Part model, mm, in its own coordinate system. Face numbers are marked on the shaded views. A direction names the side the tool comes from. Coordinates: 2 decimals unless noted, no trailing zeros. Order: outer loops, then holes, each group sorted by start corner. A loop starts at its lowest first (then second) coordinate and runs counter-clockwise, first axis right, second up. Notation, with made-up numbers: M -0.75,-36 L 46.25,-36 A7 ccw 46.25,-31 Z; hole C 60.25,35.5 d3. An arc over 180 degrees is marked long. Answer in a Markdown table with one row per item. Add a question column.
from build123d import *

# Parameters (mm, degrees)
F1_DEPTH  = 67
F2_W      = 19
F2_H      = 59.602782
F3_DEPTH  = 45
F4_W      = 19
F4_H      = 59.070988
F5_DEPTH  = 45
F7_DEPTH  = 19
F9_DEPTH  = 19
F10_W     = 28
F10_H     = 14.292508
F11_DEPTH = 66.9
F13_DEPTH = 14.4
F14_R     = 12.5
F15_DEPTH = 65.5


with BuildPart() as f1:
    # F0 (on Front) → F1 (new body)
    with BuildSketch(Plane.XZ):
        Polygon((0, 20), (0, 0), (63, 0), (63, 75), (0, 75), (0, 55), (38, 55), (38, 20), align=None)
    extrude(amount=F1_DEPTH)

    # F2 (on face) → F3 (join)
    with BuildSketch(Plane.YZ.offset(63)):
        with Locations((-49.5, 37.198609)):
            Rectangle(F2_W, F2_H)
    extrude(amount=F3_DEPTH)

    # F4 (on face) → F5 (join)
    with BuildSketch(Plane.YZ.offset(63)):
        with Locations((-16.24, 37.464506)):
            Rectangle(F4_W, F4_H)
    extrude(amount=F5_DEPTH)

    # F6 (on face) → F7 (join)
    with BuildSketch(Plane.XZ.offset(59)):
        with BuildLine():
            Line((108, 67), (108, 7.397218))
            ThreePointArc((108, 7.397218), (128.343367, 37.198609), (108, 67))
        make_face()
    extrude(amount=-F7_DEPTH)

    # F8 (on face) → F9 (join)
    with BuildSketch(Plane(origin=(0, -6.74, 0), x_dir=(-1, 0, 0), z_dir=(0, 1, 0))):
        with BuildLine():
            Line((-108, 7.929012), (-108, 67))
            ThreePointArc((-108, 67), (-127.685188, 37.464506), (-108, 7.929012))
        make_face()
    extrude(amount=-F9_DEPTH)

    # F10 (on face) → F11 (join)
    with BuildSketch(Plane.XY.offset(75)):
        with Locations((77, -32.735519)):
            Rectangle(F10_W, F10_H)
    extrude(amount=-F11_DEPTH)

    # F12 (on face) → F13 (cut)
    with BuildSketch(Plane.XZ.offset(39.881773)):
        Polygon((63, 75), (91, 66.942476), (91, 75), align=None)
    extrude(amount=-F13_DEPTH, mode=Mode.SUBTRACT)

    # F14 (on face) → F15 (cut)
    with BuildSketch(Plane.XZ.offset(59)):
        with Locations((108, 37.198609)):
            Circle(F14_R)
    extrude(amount=-F15_DEPTH, mode=Mode.SUBTRACT)


solid = f1.part
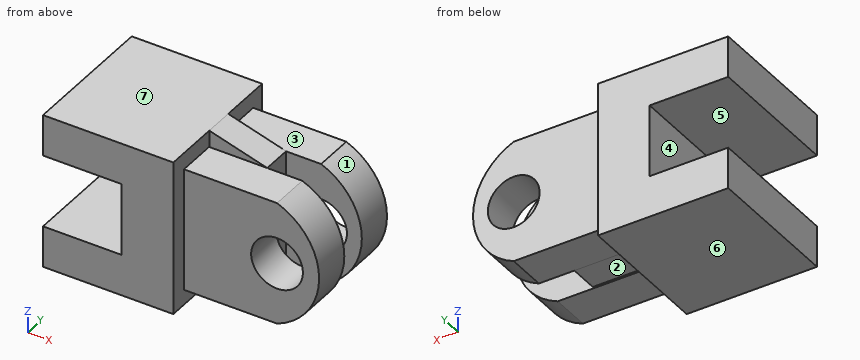
(1) Wall check: line 1 (Z direction, x = 108, y = -46.75); line 2 (Z direction, x = 108, y = -14); line 3 (Y direction, x = 118.5, z = 57). Give the ranges that are in metal, low to high.
(2) 3-axis set-ups, long thin cutter, end or side, ignore diameter. For the marked faces 1, 2, 3 and 4: which of +Z, -Z, +X, -X, +Y, -Y reach the whole face in a straight line?
(3) Slice it at B-B (z = 31). List the corners of the cut face in (x, y).
(4) Slice it at D-D (y = -35.5). List the corners of the cut face in (x, z).
(5) Pull direction Z, two halves, no side cores. Call the marked faces 5, 6 and 7: pulls with the +Z half, pulls with the -Z half, needs draft (parallel to the pull), parting line crosses it, or undercut.
(6) Slice it at A-A (x = 11.5). List the corners of the cut face in (y, z), and give its area (3 significant figures).
(7) Drop flat-ended pins along their axis: P1, Ø6.5, axis at x = 76.5, z = 71, coming from the +Y side; P2, Ø6, axis at x = 93.5, y = -14.5, coming from the +Z side; P3, Ø20, axis at y = -22, z = 43.5, coming from the +X side. Give the stop position or say it passes through.
(8) Slice it at C-C (y = -47.5). List the corners of the cut face in (x, z).
Computed:
| question | item | result |
|---|---|---|
| 1 | line 1 | z = 7.4 to 24.7, 49.7 to 67 |
| 1 | line 2 | z = 7.93 to 24.7, 49.7 to 67 |
| 1 | line 3 | y = -59 to -40, -25.74 to -6.74 |
| 2 | face 1 | +X, +Y |
| 2 | face 2 | -Z, +X |
| 2 | face 3 | +Z, +X, +Y |
| 2 | face 4 | -X, +Y, -Y |
| 3 | outline | M 38,-67 L 63,-67 L 63,-59 L 97.15,-59 L 97.15,-40 L 63,-40 L 63,-39.88 L 91,-39.88 L 91,-25.74 L 97.15,-25.74 L 97.15,-6.74 L 63,-6.74 L 63,0 L 38,0 Z; M 118.85,-59 L 127.74,-59 L 127.74,-40 L 118.85,-40 Z; M 118.85,-25.74 L 127.03,-25.74 L 127.03,-6.74 L 118.85,-6.74 Z |
| 4 | outline | M 0,0 L 63,0 L 63,8.1 L 91,8.1 L 91,66.94 L 63,75 L 0,75 L 0,55 L 38,55 L 38,20 L 0,20 Z |
| 5 | face 5 | undercut |
| 5 | face 6 | pulls with the -Z half |
| 5 | face 7 | pulls with the +Z half |
| 6 | outline | M -67,0 L 0,0 L 0,20 L -67,20 Z; M -67,55 L 0,55 L 0,75 L -67,75 Z |
| 6 | area | 2,680 mm^2 |
| 7 | P1 | stops at y = -25.59 |
| 7 | P2 | stops at z = 67 |
| 7 | P3 | stops at x = 127.69 |
| 8 | outline | M 0,0 L 63,0 L 63,7.4 L 108,7.4 A32 ccw 108,67 L 63,67 L 63,75 L 0,75 L 0,55 L 38,55 L 38,20 L 0,20 Z; hole C 108,37.2 d25 |
